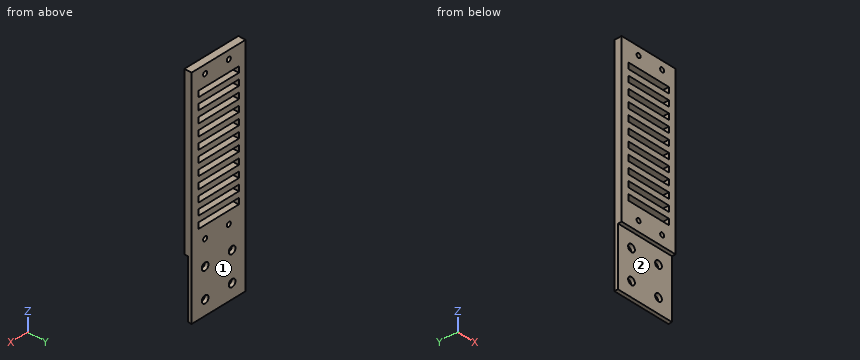
Autodesk Inventor part; units mm, degrees
ref_plane "YZ Plane" through (0, 0, 0) normal (1, 0, 0) x (0, 1, 0)
ref_plane "XZ Plane" through (0, 0, 0) normal (0, 1, 0) x (-1, 0, 0)
ref_plane "XY Plane" through (0, 0, 0) normal (0, 0, 1) x (1, 0, 0)
sketch "Sketch1" plane through (0, 0, 0) normal (0, 1, 0) x (-1, 0, 0)
  line L0 (0, 0) -> (40, 0)
  line L1 (40, 0) -> (40, -152.8)
  line L2 (40, -152.8) -> (0, -152.8)
  line L3 (0, -152.8) -> (0, 0)
  circle A0 centre (30, -122.8) radius 2.5
  circle A1 centre (30, -142.8) radius 2.5
  circle A2 centre (10, -122.8) radius 2.5
  circle A3 centre (10, -142.8) radius 2.5
  line L4 (5, -97.55) -> (35, -97.55)
  line L5 (35, -97.55) -> (35, -93.55)
  line L6 (35, -93.55) -> (5, -93.55)
  line L7 (5, -93.55) -> (5, -97.55)
  line L8 (5, -89.55) -> (35, -89.55)
  line L9 (35, -89.55) -> (35, -85.55)
  line L10 (35, -85.55) -> (5, -85.55)
  line L11 (5, -85.55) -> (5, -89.55)
  line L12 (5, -81.55) -> (35, -81.55)
  line L13 (35, -81.55) -> (35, -77.55)
  line L14 (35, -77.55) -> (5, -77.55)
  line L15 (5, -77.55) -> (5, -81.55)
  line L16 (5, -73.55) -> (35, -73.55)
  line L17 (35, -73.55) -> (35, -69.55)
  line L18 (35, -69.55) -> (5, -69.55)
  line L19 (5, -69.55) -> (5, -73.55)
  line L20 (5, -65.55) -> (35, -65.55)
  line L21 (35, -65.55) -> (35, -61.55)
  line L22 (35, -61.55) -> (5, -61.55)
  line L23 (5, -61.55) -> (5, -65.55)
  line L24 (5, -57.55) -> (35, -57.55)
  line L25 (35, -57.55) -> (35, -53.55)
  line L26 (35, -53.55) -> (5, -53.55)
  line L27 (5, -53.55) -> (5, -57.55)
  line L28 (5, -49.55) -> (35, -49.55)
  line L29 (35, -49.55) -> (35, -45.55)
  line L30 (35, -45.55) -> (5, -45.55)
  line L31 (5, -45.55) -> (5, -49.55)
  line L32 (5, -41.55) -> (35, -41.55)
  line L33 (35, -41.55) -> (35, -37.55)
  line L34 (35, -37.55) -> (5, -37.55)
  line L35 (5, -37.55) -> (5, -41.55)
  line L36 (5, -33.55) -> (35, -33.55)
  line L37 (35, -33.55) -> (35, -29.55)
  line L38 (35, -29.55) -> (5, -29.55)
  line L39 (5, -29.55) -> (5, -33.55)
  line L40 (5, -25.55) -> (35, -25.55)
  line L41 (35, -25.55) -> (35, -21.55)
  line L42 (35, -21.55) -> (5, -21.55)
  line L43 (5, -21.55) -> (5, -25.55)
  line L44 (5, -17.55) -> (35, -17.55)
  line L45 (35, -17.55) -> (35, -13.55)
  line L46 (35, -13.55) -> (5, -13.55)
  line L47 (5, -13.55) -> (5, -17.55)
  dimension "d0" = 40
  dimension "d1" = 152.8
  dimension "d2" = 5
  dimension "d3" = 5
  dimension "d4" = 5
  dimension "d5" = 5
  dimension "d6" = 10
  dimension "d7" = 0
  dimension "d8" = 20
  dimension "d11" = 30
  dimension "d12" = 20
  dimension "d13" = 30
  dimension "d14" = 10
  dimension "d15" = 0
  dimension "d16" = 30
  dimension "d18" = 55.25
  dimension "d31" = 30
  dimension "d33" = 30
  dimension "d35" = 30
  dimension "d37" = 30
  dimension "d39" = 30
  dimension "d41" = 30
  dimension "d43" = 30
  dimension "d45" = 30
  dimension "d47" = 30
  dimension "d49" = 30
extrude "Extrusion1" add sketch "Sketch1" along normal blind 5
sketch "Sketch2" plane through (0, 5, 0) normal (0, 1, 0) x (1, 0, 0)
  line L0 (-5, 17.55) -> (-5, 13.55)
  line L1 (-5, 13.55) -> (-35, 13.55)
  line L2 (-35, 13.55) -> (-35, 17.55)
  line L3 (-35, 17.55) -> (-5, 17.55)
  line L4 (-5, 25.55) -> (-5, 21.55)
  line L5 (-5, 21.55) -> (-35, 21.55)
  line L6 (-35, 21.55) -> (-35, 25.55)
  line L7 (-35, 25.55) -> (-5, 25.55)
  line L8 (-5, 33.55) -> (-5, 29.55)
  line L9 (-5, 29.55) -> (-35, 29.55)
  line L10 (-35, 29.55) -> (-35, 33.55)
  line L11 (-35, 33.55) -> (-5, 33.55)
  line L12 (-5, 41.55) -> (-5, 37.55)
  line L13 (-5, 37.55) -> (-35, 37.55)
  line L14 (-35, 37.55) -> (-35, 41.55)
  line L15 (-35, 41.55) -> (-5, 41.55)
  line L16 (-5, 49.55) -> (-5, 45.55)
  line L17 (-5, 45.55) -> (-35, 45.55)
  line L18 (-35, 45.55) -> (-35, 49.55)
  line L19 (-35, 49.55) -> (-5, 49.55)
  line L20 (-5, 57.55) -> (-5, 53.55)
  line L21 (-5, 53.55) -> (-35, 53.55)
  line L22 (-35, 53.55) -> (-35, 57.55)
  line L23 (-35, 57.55) -> (-5, 57.55)
  line L24 (-5, 65.55) -> (-5, 61.55)
  line L25 (-5, 61.55) -> (-35, 61.55)
  line L26 (-35, 61.55) -> (-35, 65.55)
  line L27 (-35, 65.55) -> (-5, 65.55)
  line L28 (-5, 73.55) -> (-5, 69.55)
  line L29 (-5, 69.55) -> (-35, 69.55)
  line L30 (-35, 69.55) -> (-35, 73.55)
  line L31 (-35, 73.55) -> (-5, 73.55)
  line L32 (-5, 81.55) -> (-5, 77.55)
  line L33 (-5, 77.55) -> (-35, 77.55)
  line L34 (-35, 77.55) -> (-35, 81.55)
  line L35 (-35, 81.55) -> (-5, 81.55)
  line L36 (-5, 89.55) -> (-5, 85.55)
  line L37 (-5, 85.55) -> (-35, 85.55)
  line L38 (-35, 85.55) -> (-35, 89.55)
  line L39 (-35, 89.55) -> (-5, 89.55)
  line L40 (-5, 97.55) -> (-5, 93.55)
  line L41 (-5, 93.55) -> (-35, 93.55)
  line L42 (-35, 93.55) -> (-35, 97.55)
  line L43 (-35, 97.55) -> (-5, 97.55)
  circle A0 centre (-10, 142.8) radius 2.5
  circle A1 centre (-10, 122.8) radius 2.5
  circle A2 centre (-30, 142.8) radius 2.5
  circle A3 centre (-30, 122.8) radius 2.5
  line L44 (-40, 0) -> (0, 0)
  line L45 (0, 0) -> (0, 152.8)
  line L46 (0, 152.8) -> (-40, 152.8)
  line L47 (-40, 152.8) -> (-40, 0)
  circle A4 centre (-27.5, 5.625) radius 1.5
  circle A5 centre (-10, 5.625) radius 1.5
  circle A6 centre (-27.5, 105.925) radius 1.5
  circle A7 centre (-10, 105.925) radius 1.5
  dimension "d53" = 3
  dimension "d54" = 3
  dimension "d55" = 3
  dimension "d56" = 3
  dimension "d57" = 12.5
  dimension "d58" = 10
  dimension "d59" = 12.5
  dimension "d60" = 10
  dimension "d61" = 5.625
  dimension "d62" = 5.625
  dimension "d63" = 46.875
  dimension "d64" = 46.875
extrude "Extrusion2" cut sketch "Sketch2" against normal blind 5 contours A4 | A5 | A6 | A7
sketch "Sketch3" plane through (0, 0, 0) normal (0, -1, 0) x (1, 0, 0)
  circle A0 centre (-27.5, -105.925) radius 1.5
  circle A1 centre (-27.5, -5.625) radius 1.5
  circle A2 centre (-10, -5.625) radius 1.5
  circle A3 centre (-10, -105.925) radius 1.5
  line L0 (-5, -13.55) -> (-5, -17.55)
  line L1 (-5, -17.55) -> (-35, -17.55)
  line L2 (-35, -17.55) -> (-35, -13.55)
  line L3 (-35, -13.55) -> (-5, -13.55)
  line L4 (-5, -21.55) -> (-5, -25.55)
  line L5 (-5, -25.55) -> (-35, -25.55)
  line L6 (-35, -25.55) -> (-35, -21.55)
  line L7 (-35, -21.55) -> (-5, -21.55)
  line L8 (-5, -29.55) -> (-5, -33.55)
  line L9 (-5, -33.55) -> (-35, -33.55)
  line L10 (-35, -33.55) -> (-35, -29.55)
  line L11 (-35, -29.55) -> (-5, -29.55)
  line L12 (-5, -37.55) -> (-5, -41.55)
  line L13 (-5, -41.55) -> (-35, -41.55)
  line L14 (-35, -41.55) -> (-35, -37.55)
  line L15 (-35, -37.55) -> (-5, -37.55)
  line L16 (-5, -45.55) -> (-5, -49.55)
  line L17 (-5, -49.55) -> (-35, -49.55)
  line L18 (-35, -49.55) -> (-35, -45.55)
  line L19 (-35, -45.55) -> (-5, -45.55)
  line L20 (-5, -53.55) -> (-5, -57.55)
  line L21 (-5, -57.55) -> (-35, -57.55)
  line L22 (-35, -57.55) -> (-35, -53.55)
  line L23 (-35, -53.55) -> (-5, -53.55)
  line L24 (-5, -61.55) -> (-5, -65.55)
  line L25 (-5, -65.55) -> (-35, -65.55)
  line L26 (-35, -65.55) -> (-35, -61.55)
  line L27 (-35, -61.55) -> (-5, -61.55)
  line L28 (-5, -69.55) -> (-5, -73.55)
  line L29 (-5, -73.55) -> (-35, -73.55)
  line L30 (-35, -73.55) -> (-35, -69.55)
  line L31 (-35, -69.55) -> (-5, -69.55)
  line L32 (-5, -77.55) -> (-5, -81.55)
  line L33 (-5, -81.55) -> (-35, -81.55)
  line L34 (-35, -81.55) -> (-35, -77.55)
  line L35 (-35, -77.55) -> (-5, -77.55)
  line L36 (-5, -85.55) -> (-5, -89.55)
  line L37 (-5, -89.55) -> (-35, -89.55)
  line L38 (-35, -89.55) -> (-35, -85.55)
  line L39 (-35, -85.55) -> (-5, -85.55)
  line L40 (-5, -93.55) -> (-5, -97.55)
  line L41 (-5, -97.55) -> (-35, -97.55)
  line L42 (-35, -97.55) -> (-35, -93.55)
  line L43 (-35, -93.55) -> (-5, -93.55)
  circle A4 centre (-10, -142.8) radius 2.5
  circle A5 centre (-10, -122.8) radius 2.5
  circle A6 centre (-30, -142.8) radius 2.5
  circle A7 centre (-30, -122.8) radius 2.5
  line L44 (0, 0) -> (-40, 0)
  line L45 (-40, 0) -> (-40, -152.8)
  line L46 (-40, -152.8) -> (0, -152.8)
  line L47 (0, -152.8) -> (0, 0)
  line L48 (0, 0) -> (0, -152.8)
  line L49 (-40, -152.8) -> (0, -152.8)
  line L50 (0, -152.8) -> (0, -112.8)
  line L51 (0, -112.8) -> (-40, -112.8)
  line L52 (-40, -112.8) -> (-40, -152.8)
  dimension "d67" = 40
extrude "Extrusion3" cut sketch "Sketch3" against normal blind 2.5 contours L47 L46 L45 L51
properties part number "Base Right Front Panel"
Read the model definition and answer for the solid it produces. Units are mm, in the model's axes. Face numbers are marked on the shaded views. A direction names the side the tool comes from. Coordinates: 2 decimals unless noted, no trailing zeros. Order: outer loops, then holes, each group sorted by start corner. A loop starts at its lowest first (then second) coordinate and runs counter-clockwise, first axis right, second up. Notation, with made-up numbers: M -39,0 L 18,0 A23 cw 18,9 Z; hole C 55,73.5 d2. An arc over 180 degrees is marked long. Put each result on its own line as item: value. Start each with the question number.
Item 1: Given pin 1 Ø6 at (x, z) = (-30, -122.8) entering from -Y, flat-ended and moving along its own axis, determine where the tip first touches the part or whether it passes through.
Item 2: For the marked faces 1 and 2, determine the directions among +Z, -Z, +X, -X, +Y, -Y from which every point of the face is accessible in a straight line to the end or side of a thin tool.
Item 3: Section B-B, the plane x = -10 is taken. Count the separate pieces of the cut face and the enclosed holes in it, plus the area to 3 significant figures.
Item 4: Section A-A, the plane z = -142.8 is taken. Determine the outline of the cut face in (x, y), plus the area to 3 significant figures.
Item 5: Consider probe 1 along X at (y, z) = (1.1, -14); probe 2 along Y at (x, z) = (-22.5, -114.5); probe 3 along Z at (x, y) = (-3.5, 1.65). Determine where each line is inside the solid, lowest interval first. Write a range as [from, to].
Computed:
1. pin 1: stops at y = 2.5
2. face 1: +Z, -Z, +X, -X, +Y
2. face 2: -Z, +X, -X, -Y
3. separate pieces: 16
3. enclosed holes: 0
3. area: 389 mm2
4. outline: M -40,2.5 L -32.5,2.5 L -32.5,5 L -40,5 Z; M -27.5,2.5 L -12.5,2.5 L -12.5,5 L -27.5,5 Z; M -7.5,2.5 L 0,2.5 L 0,5 L -7.5,5 Z
4. area: 75.0 mm2
5. probe 1: x = [-40, -35], [-5, 0]
5. probe 2: y = [2.5, 5]
5. probe 3: z = [-112.8, 0]
